Solid Edge part; units mm, degrees
sketch "Sketch1" plane through (0, 0, 0) normal (0, -1, 0) x (1, 0, 0)
  line L0 (-15, 10) -> (15, 10)
  line L1 (15, 10) -> (15, -10)
  line L2 (15, -10) -> (-15, -10)
  line L3 (-15, -10) -> (-15, 10)
  dimension "D1" = 15
  dimension "D2" = 15
extrude "Protrusion1" add sketch "Sketch1" along normal mid plane 33
sketch "Sketch2" plane through (0, -16.5, 0) normal (0, -1, 0) x (1, 0, 0)
  line L0 (-25, 17.5) -> (25, 17.5)
  line L1 (25, 17.5) -> (25, -17.5)
  line L2 (25, -17.5) -> (-25, -17.5)
  line L3 (-25, -17.5) -> (-25, 17.5)
  dimension "D1" = 25
  dimension "D2" = 25
extrude "Ausprägung_2" add sketch "Sketch2" along normal blind 4
sketch "Sketch3" plane through (0, -20.5, 0) normal (0, -1, 0) x (1, 0, 0)
  line L0 (-6.75, 3) -> (6.75, 3)
  line L1 (6.75, 3) -> (6.75, -3)
  line L2 (6.75, -3) -> (-6.75, -3)
  line L3 (-6.75, -3) -> (-6.75, 3)
  dimension "D1" = 6.75
  dimension "D2" = 6.75
extrude "Ausschnitt_1" cut sketch "Sketch3" against normal blind 9
sketch "Sketch4" plane through (0, -11.5, 0) normal (0, -1, 0) x (1, 0, 0)
  line L0 (-8.25, 5.5) -> (8.25, 5.5)
  line L1 (8.25, 5.5) -> (8.25, -5.5)
  line L2 (8.25, -5.5) -> (-8.25, -5.5)
  line L3 (-8.25, -5.5) -> (-8.25, 5.5)
  dimension "D1" = 8.25
  dimension "D2" = 8.25
extrude "Ausschnitt_2" cut sketch "Sketch4" against normal blind 23
sketch "Sketch5" plane through (0, 16.5, 0) normal (0, 1, 0) x (-1, 0, 0)
  line L0 (6.25, 5.5) -> (6.25, -5.5)
  line L1 (6.25, -5.5) -> (-6.25, -5.5)
  line L2 (-6.25, -5.5) -> (-6.25, 5.5)
  line L3 (-6.25, 5.5) -> (6.25, 5.5)
  dimension "D1" = 6.25
  dimension "D2" = 6.25
extrude "Ausschnitt_3" cut sketch "Sketch5" against normal blind 5
sketch "Sketch6" plane through (0, -20.5, 0) normal (0, -1, 0) x (1, 0, 0)
  line L0 (-37.3753, 23.8002) -> (37.3753, 23.8002)
  line L1 (37.3753, 23.8002) -> (37.3753, 0)
  line L2 (37.3753, 0) -> (-37.3753, 0)
  line L3 (-37.3753, 0) -> (-37.3753, 23.8002)
extrude "Ausschnitt_4" cut sketch "Sketch6" against normal blind 187.325
hole "Bohrung_1" at (20, -20.5, -12.5) direction (0, 1, 0) diameter 3.5 end up to next countersink diameter 5.5 countersink angle 90
hole "Hole1" at (-20, -20.5, -12.5) direction (0, 1, 0) diameter 3.5 end up to next countersink diameter 5.5 countersink angle 90
hole "Bohrung_3" at (11.5, -11.5, 0) direction (0, 0, -1) diameter 2.5 end through all
hole "Hole2" at (11.5, 11.5, 0) direction (0, 0, -1) diameter 2.5 end through all
hole "Bohrung_5" at (-11.5, 11.5, -10) direction (0, 0, 1) diameter 3.5 end up to next countersink diameter 5.5 countersink angle 90
hole "Hole3" at (-11.5, -11.5, -10) direction (0, 0, 1) diameter 3.5 end up to next countersink diameter 5.5 countersink angle 90
fillet "Verrundung_2" radius 2 3 edges at (25, -20.5, -8.75) (0, -20.5, -17.5) (-25, -20.5, -8.75)
fillet "Verrundung_3" radius 0.5 5 edges at (15, 0, -10) (0, 16.5, -10) (-15, 0, -10) (-15, 16.5, -5) (15, 16.5, -5)
Could you check a few things on this model? Use its own coordinates, in mm. A direction names the side the tool comes from. Coordinates: 2 decimals unless noted, no trailing zeros. Write each loop counter-clockwise with the first axis right and the second up, starting at its lowest first coordinate (ties: lowest second). Pieces come first, ordered by that corner, then holes. Notation, with made-up numbers: (-10, -16) -> (2, -16) arc R24 cw to (2, -5) -> close; hole circle Ø1 at (21, 42.25). An arc over 180 degrees is marked (long way). Return JSON: item names as keys, results as strings.
(1) Imagine slicing it at B-B, the plane z = -12.5. Please give me the cut outline in (x, y).
Numbers:
{"outline": "(-25, -18.5) arc R2 ccw to (-23, -20.5) -> (-22.75, -20.5) -> (-21.75, -19.5) -> (-21.75, -16.5) -> (-25, -16.5) -> close; (-18.25, -19.5) -> (-17.25, -20.5) -> (17.25, -20.5) -> (18.25, -19.5) -> (18.25, -16.5) -> (-18.25, -16.5) -> close; (21.75, -19.5) -> (22.75, -20.5) -> (23, -20.5) arc R2 ccw to (25, -18.5) -> (25, -16.5) -> (21.75, -16.5) -> close"}
(2) Imagine slicing it at A-A, the plane x = -20. Please give me the cut outline in (y, z).
Numbers:
{"outline": "(-20.5, -15.5) arc R2 ccw to (-18.5, -17.5) -> (-16.5, -17.5) -> (-16.5, -14.25) -> (-19.5, -14.25) -> (-20.5, -15.25) -> close; (-20.5, -9.75) -> (-19.5, -10.75) -> (-16.5, -10.75) -> (-16.5, 0) -> (-20.5, 0) -> close"}
(3) Which directions (+Z, -Z, +X, -X, +Y, -Y) give clear straight access to the entire face, cutting with the end or side of a thin tool? Please do faces 4 (the flat face through (0, -11.5, -4)), 5 (the flat face through (0, -16.5, -11)), 6 (the flat face through (-15, 0, -5)), 7 (the flat face through (15, 0, -5)).
Numbers:
{"face 4": "+Z", "face 5": "-Z, +Y", "face 6": "+Z, -Z, -X, +Y", "face 7": "+Z, -Z, +X, +Y"}
(4) Imagine slicing it at D-D, the plane x = -2. Please give me the cut outline in (y, z), then the cut area to 3 significant figures.
Numbers:
{"outline": "(-20.5, -15.5) arc R2 ccw to (-18.5, -17.5) -> (-16.5, -17.5) -> (-16.5, -10) -> (16, -10) arc R0.5 ccw to (16.5, -9.5) -> (16.5, -5.5) -> (-11.5, -5.5) -> (-11.5, -3) -> (-20.5, -3) -> close", "area": "218 mm2"}
(5) I need wall thicknesses on L1, parallel to Y at x = 11.5, z = -2.5; L2, parallel to X at y = -17.6, z = -12.5; L3, parallel to Y at x = -11.5, z = -4.5. Which ranges of each line are inside material? Lowest first, please.
Numbers:
{"L1": "y = -20.5 to -12.75, -10.25 to 10.25, 12.75 to 16.5", "L2": "x = -25 to -21.75, -18.25 to 18.25, 21.75 to 25", "L3": "y = -20.5 to -13.25, -9.75 to 9.75, 13.25 to 16.5"}
(6) I'm going to push flat-ended pins straight in: pin 1 (1.6 mm diameter, centred on y = 5.5, z = -4, fed in from -X); pin 2 (2 mm diameter, centred on x = -11.5, y = 11.5, fed in from -Z); pin 3 (6 mm diameter, centred on x = 12.5, y = 0.5, fed in from -Z); pin 4 (8 mm diameter, centred on y = -9, z = -4, fed in from +X). Where does each tip first touch, or does it pass through?
Numbers:
{"pin 1": "stops at x = -15", "pin 2": "passes through", "pin 3": "stops at z = -10", "pin 4": "stops at x = 15"}
(7) Imagine slicing it at C-C, the plane y = 2.5. Please give me the cut outline in (x, z).
Numbers:
{"outline": "(-15, -9.5) arc R0.5 ccw to (-14.5, -10) -> (14.5, -10) arc R0.5 ccw to (15, -9.5) -> (15, 0) -> (8.25, 0) -> (8.25, -5.5) -> (-8.25, -5.5) -> (-8.25, 0) -> (-15, 0) -> close"}
(8) We'd pull the mould along Y, two halves only. Please class faces 1 (the cylindrical face through (-10, 12.4, -4.6)), 2 (the flat face through (0, -20.5, -8)), 3 (the flat face through (6.25, 14, -3)): +Y half, -Y half, draft (parallel to the pull), parting line (faces both ways), or undercut.
Numbers:
{"face 1": "undercut", "face 2": "-Y half", "face 3": "draft"}
